Part model, mm, in its own coordinate system. A direction names the side the tool comes from. Coordinates: 2 decimals unless noted, no trailing zeros. Loops run counter-clockwise (first coordinate to the right, second up) from the corner with the lowest first, then second, coordinate; pieces in that order, holes last. Notation, with made-up numbers: (59.25, 6.25) - (118.25, 6.25) arc R21 cw to (118.25, 20.25) - close; hole circle Ø8 at (89.25, -18.75). An arc over 180 degrees is marked (long way). Use a Markdown table: item, result. Add a question column.
1) Band-saw the part on A-A (y = 8.5). Give the cut face in (x, z), plus the area to 3 significant figures.
2) Band-saw the part on D-D (x = 0). Give the cut face in (y, z).
3) Tool access for faces 1 (the face through (-0.8, -6.094, -0.167)), 2 (the face through (0, 6, -11.906)): list every direction of +Z, -Z, +X, -X, +Y, -Y with a clear straight run to the whole face (end or side of a thin tool).
4) Probe probe 1 along Z at (x, y) = (5.75, 12); probe 2 along Y at (x, z) = (-0.25, -7.5); probe 3 along Y at (x, z) = (3.5, -3.5). List the from-to ranges inside material, lowest first. Write a range as [from, to].
5) Pull direction Y, two halves, no side cores. Call faces 3 (the face through (0, 14.288, 0)), 4 (the face through (0, 6, 11.906)), 5 (the face through (0, 17.462, 0)): +Y half, -Y half, draft (parallel to the pull), parting line (faces both ways), or undercut.
6) Band-saw the part on C-C (x = -3.5). Give the cut face in (y, z), plus the area to 3 significant figures.
7) Drop a flat-ended pin along its axis: P1, Ø1.5, axis at y = 1.5, z = 6.5, coming from the -X side. Give the stop position or say it passes through.
8) Band-saw the part on B-B (z = -4.5). Give the cut face in (x, y), plus the area to 3 significant figures.
from build123d import *

# Parameters (mm, degrees)
SKETCH1_R             = 6.1468
BOSS_EXTRUDE1_DEPTH   = 8.73125
SKETCH1_W             = 12.2936
SKETCH1_H             = 3.175
BOSS_EXTRUDE1_2_DEPTH = 8.73125
BOSS_EXTRUDE2_START   = 3.175
BOSS_EXTRUDE2_DEPTH   = 3.175


with BuildPart() as part:
    # Sketch1 → Boss-Extrude1 (new, symmetric)
    with BuildSketch(Plane.XY):
        Circle(SKETCH1_R)
    extrude(amount=BOSS_EXTRUDE1_DEPTH, both=True)



with BuildPart() as body_2:
    # Sketch1 → Boss-Extrude1 2 (new, symmetric)
    with BuildSketch(Plane.XY):
        with Locations((0, 15.875)):
            Rectangle(SKETCH1_W, SKETCH1_H)
    extrude(amount=BOSS_EXTRUDE1_2_DEPTH, both=True)


with BuildPart() as part_1:
    add(part.part)

    add(body_2.part)  # Boss-Extrude2 merges body 2
    # Sketch2 → Boss-Extrude2 (add)
    with BuildSketch(Plane.XY.offset(8.73125).offset(BOSS_EXTRUDE2_START)):
        with BuildLine():
            Line((-6.1468, 0), (-6.1468, 17.4625))
            Line((-6.1468, 17.4625), (6.1468, 17.4625))
            Line((6.1468, 17.4625), (6.1468, 0))
            ThreePointArc((6.1468, 0), (0, -6.1468), (-6.1468, 0))
        make_face()
    boss_extrude2 = extrude(amount=-BOSS_EXTRUDE2_DEPTH)

    # Mirror1: Boss-Extrude2 across plane
    add(boss_extrude2.mirror(Plane.XY))


solid = part_1.part
Answer block:
| question | item | result |
|---|---|---|
| 1 | outline | (-6.15, -11.91) - (6.15, -11.91) - (6.15, -8.73) - (-6.15, -8.73) - close; (-6.15, 8.73) - (6.15, 8.73) - (6.15, 11.91) - (-6.15, 11.91) - close |
| 1 | area | 78.1 mm2 |
| 2 | outline | (-6.15, -11.91) - (17.46, -11.91) - (17.46, 11.91) - (-6.15, 11.91) - close; hole (6.15, -8.73) - (14.29, -8.73) - (14.29, 8.73) - (6.15, 8.73) - close |
| 3 | face 1 | none |
| 3 | face 2 | -Z, +X, -X, +Y, -Y |
| 4 | probe 1 | [-11.91, -8.73], [8.73, 11.91] |
| 4 | probe 2 | [-6.14, 6.14], [14.29, 17.46] |
| 4 | probe 3 | [-5.05, 5.05], [14.29, 17.46] |
| 5 | face 3 | undercut |
| 5 | face 4 | draft |
| 5 | face 5 | +Y half |
| 6 | outline | (-5.05, -11.91) - (17.46, -11.91) - (17.46, 11.91) - (-5.05, 11.91) - close; hole (5.05, -8.73) - (14.29, -8.73) - (14.29, 8.73) - (5.05, 8.73) - close |
| 6 | area | 375 mm2 |
| 7 | P1 | x = -6.1 |
| 8 | outline | circle Ø12.29 at (0, 0); (-6.15, 14.29) - (6.15, 14.29) - (6.15, 17.46) - (-6.15, 17.46) - close |
| 8 | area | 158 mm2 |
